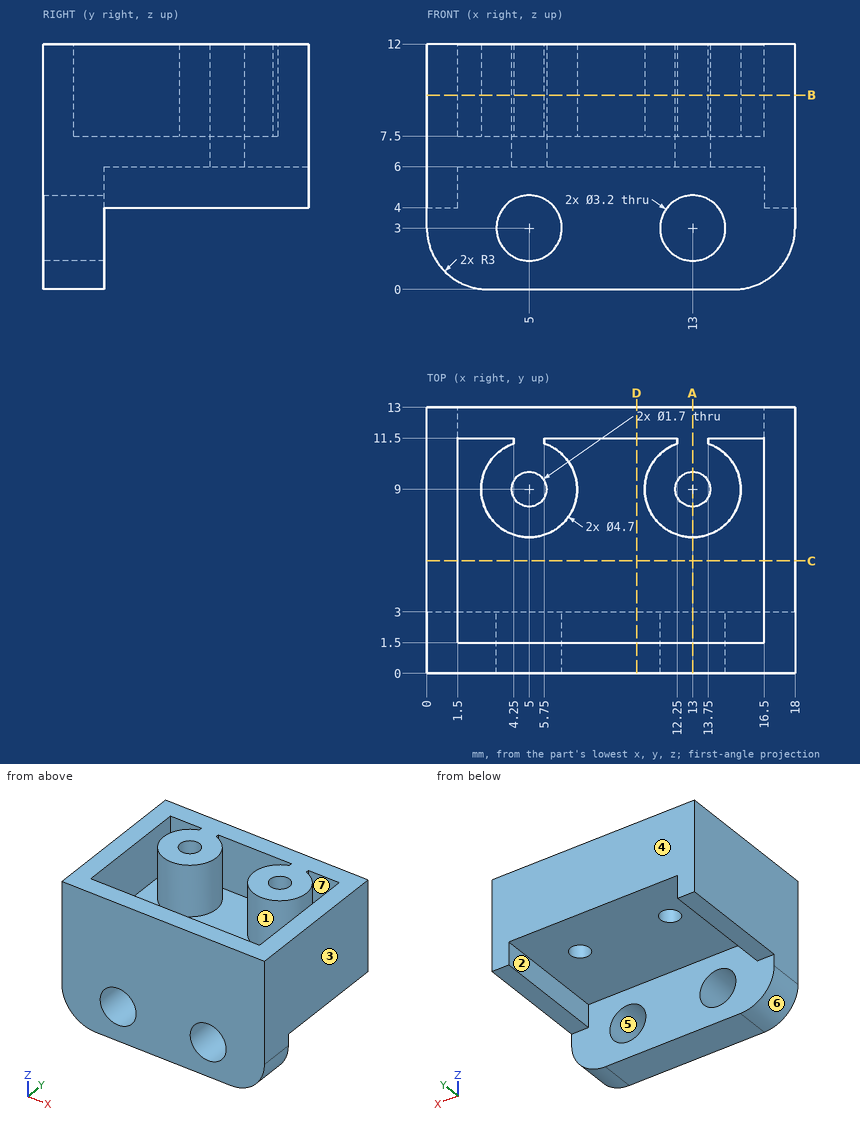
Drawing for the job (mm, zero at the part's lowest x, y, z). A direction names the side the tool comes from. Round coordinates to 2 decimals unless told otherwise and drop trailing zeros. Order: outer loops, then holes, each group sorted by start corner. A loop starts at its lowest first (then second) coordinate and runs counter-clockwise, first axis right, second up.
Item 1: Saw through at B-B on z = 9.5. Write the cut outline in (x, y), then the cut area to 3 significant figures.
Item 2: Tool access for the marked faces 1, 2 and 3: list every direction of +Z, -Z, +X, -X, +Y, -Y with a clear straight run to the whole face (end or side of a thin tool).
Item 3: Saw through at A-A on x = 13. Write the cut outline in (y, z).
Item 4: Mould opens along X. For the marked faces 4, 5, 6 and 7 say: pulls with the +X half, pulls with the -X half, needs draft (parallel to the pull), parting line crosses it, or undercut.
Item 5: Saw through at D-D on x = 10.25. Write the cut outline in (y, z), then the cut area to 3 significant figures.
Item 6: Pin check, flat tips, straight feed: pin 1 (4 mm diameter, centred on y = 8, z = 3.5, fed in from -X); pin 2 (1.5 mm diameter, centred on x = 2.5, y = 6.5, fed in from +Z); pin 3 (1.9 mm diameter, centred on x = 13, z = 3, fed in from -Y); pin 4 (1.2 mm diameter, centred on x = 0.5, y = 8, fed in from -Z). Stop position of each tip, or through.
Item 7: Saw through at C-C on y = 5.5. Write the cut outline in (x, z).
Item 8: Probe line 1 along X through (y, z) = (1.5, 3); line 2 along Y through (x, z) = (15.75, 10.25); line 3 along X through (y, z) = (7.75, 4.75). List the from-to ranges inside material, lowest first.
Reported:
1. outline: (0, 0) - (18, 0) - (18, 13) - (0, 13) - close; hole (1.5, 1.5) - (16.5, 1.5) - (16.5, 11.5) - (13.75, 11.5) - (13.75, 11.23) arc R2.35 cw (long way) to (12.25, 11.23) - (12.25, 11.5) - (5.75, 11.5) - (5.75, 11.23) arc R2.35 cw (long way) to (4.25, 11.23) - (4.25, 11.5) - (1.5, 11.5) - close; hole circle Ø1.7 at (5, 9); hole circle Ø1.7 at (13, 9)
1. area: 115 mm2
2. face 1: +Z
2. face 2: -Z, +Y
2. face 3: +Z, -Z, +X, +Y, -Y
3. outline: (0, 0) - (3, 0) - (3, 1.4) - (0, 1.4) - close; (0, 4.6) - (3, 4.6) - (3, 6) - (8.15, 6) - (8.15, 12) - (6.65, 12) - (6.65, 7.5) - (1.5, 7.5) - (1.5, 12) - (0, 12) - close; (9.85, 6) - (13, 6) - (13, 12) - (9.85, 12) - close
4. face 4: needs draft
4. face 5: undercut
4. face 6: pulls with the -X half
4. face 7: undercut
5. outline: (0, 0) - (3, 0) - (3, 6) - (13, 6) - (13, 12) - (11.5, 12) - (11.5, 7.5) - (1.5, 7.5) - (1.5, 12) - (0, 12) - close
5. area: 51.0 mm2
6. pin 1: stops at x = 0
6. pin 2: stops at z = 7.5
6. pin 3: passes through
6. pin 4: stops at z = 4
7. outline: (0, 4) - (1.5, 4) - (1.5, 6) - (16.5, 6) - (16.5, 4) - (18, 4) - (18, 12) - (16.5, 12) - (16.5, 7.5) - (1.5, 7.5) - (1.5, 12) - (0, 12) - close
8. line 1: x = 0 to 3.4, 6.6 to 11.4, 14.6 to 18
8. line 2: y = 0 to 1.5, 11.5 to 13
8. line 3: x = 0 to 1.5, 16.5 to 18
